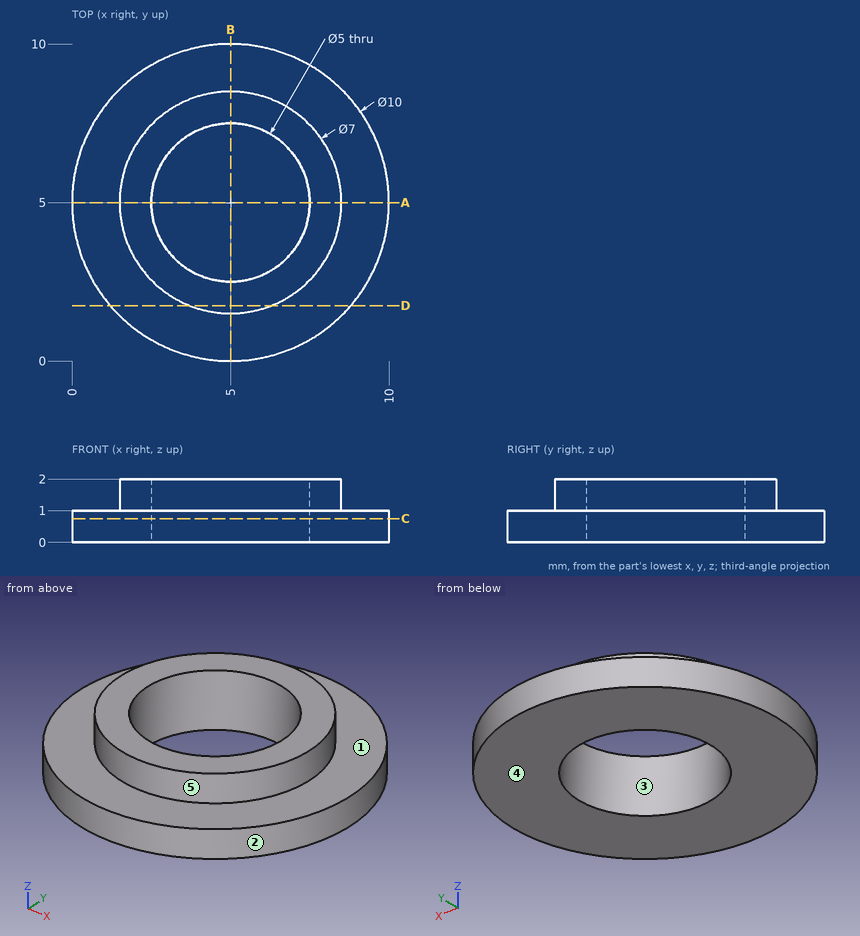
For this review, use the dimensioned drawing (mm, ordinates from the lowest corner) and the shaded views. A direction names the side the tool comes from. Coordinates: 2 decimals unless noted, no trailing zeros. Write each loop counter-clockwise with the first axis right and the second up, starting at its lowest first coordinate (ties: lowest second). Pieces come first, ordered by that corner, then holes. Notation, with made-up numbers: (47.25, 81.5) -> (53.25, 81.5) arc R7 cw to (53.25, 85.5) -> close; hole circle Ø9 at (31, 57.5). An arc over 180 degrees is marked (long way). Write each question's results on one line, items separated by ' | '. Start each with the question number.
(1) The part is to be moulded in two halves that separate along Y. For the marked faces 1, 2 and 3, say which applies: pulls with the +Y half, pulls with the -Y half, needs draft (parallel to the pull), parting line crosses it, or undercut.
(2) For line 1 along Y through (x, z) = (5, 1.2); line 2 along Z through (x, y) = (0.5, 6.5); line 3 along Y through (x, z) = (5, 0.65), list the stretches that pass through material, from the lowest coordinate up. Write a range as from..to.
(3) Clearance check with a flat-ended pin moving along its axis: P1, Ø3, axis at x = 5, y = 5, coming from the +Z side. State where the tip first meets the part, or that it passes through.
(4) Take a section at A-A on y = 5. Write out the cut boundary in (x, z), and give its area (3 significant figures).
(5) Take a section at D-D on y = 1.75. Write out the cut boundary in (x, z), and give its area (3 significant figures).
(6) Take a section at C-C on z = 0.75. Write out the cut boundary in (x, y), and give its area (3 significant figures).
(7) Tool access review of the marked faces 4 and 5: name each direction out of +Z, -Z, +X, -X, +Y, -Y from which nothing blocks a thin tool from reaching the whole face with its end or side.
Results found:
1) face 1: needs draft | face 2: parting line crosses it | face 3: undercut
2) line 1: y = 1.5..2.5, 7.5..8.5 | line 2: z = 0..1 | line 3: y = 0..2.5, 7.5..10
3) P1: passes through
4) outline: (0, 0) -> (2.5, 0) -> (2.5, 2) -> (1.5, 2) -> (1.5, 1) -> (0, 1) -> close; (7.5, 0) -> (10, 0) -> (10, 1) -> (8.5, 1) -> (8.5, 2) -> (7.5, 2) -> close | area: 7.00 mm2
5) outline: (1.2, 0) -> (8.8, 0) -> (8.8, 1) -> (6.3, 1) -> (6.3, 2) -> (3.7, 2) -> (3.7, 1) -> (1.2, 1) -> close | area: 10.2 mm2
6) outline: circle Ø10 at (5, 5); hole circle Ø5 at (5, 5) | area: 58.9 mm2
7) face 4: -Z, +X, -X, +Y, -Y | face 5: +Z
